```python
from build123d import *

# Parameters (mm, degrees)
F0_W     = 19.97
F0_H     = 100
F1_DEPTH = 0.6
F2_R     = 9.5
F3_R     = 2
F4_DEPTH = 0.601


with BuildPart() as f1:
    # F0 (on Front) → F1 (new body)
    with BuildSketch(Plane.XZ):
        with Locations((0, 50)):
            Rectangle(F0_W, F0_H)
        with Locations((0, -50)):
            Rectangle(F0_W, F0_H)
    extrude(amount=F1_DEPTH)

    # F2
    f2_edges = [f1.edges().sort_by_distance(p)[0] for p in [
        (9.985, -0.3, 100),
        (-9.985, -0.3, 100),
        (9.985, -0.3, -100),
        (-9.985, -0.3, -100),
    ]]
    fillet(f2_edges, radius=F2_R)

    # F3 (on face) → F4 (cut, through all)
    with BuildSketch(Plane.XZ.offset(0.6)):
        with Locations((0, 90.5)):
            Circle(F3_R)
        with Locations((0, -90.5)):
            Circle(F3_R)
    extrude(amount=-F4_DEPTH, mode=Mode.SUBTRACT)


solid = f1.part
```
Could you check a few things on this model? Use its own coordinates, in mm. Coordinates: 2 decimals unless noted, no trailing zeros. Order: outer loops, then holes, each group sorted by start corner. A loop starts at its lowest first (then second) coordinate and runs counter-clockwise, first axis right, second up. Notation, with made-up numbers: M 77.25,38 L 106.25,38 A20 ccw 106.25,72 Z; hole C 80.25,65 d11. An arc over 180 degrees is marked long. Use a Markdown table: item, result. Add a question column.
Q1. I want a section at B-B on x = -6. List the corners of the cut face in (y, z) for me, then the cut area to 3 significant figures.
Q2. I want a section at A-A on y = -0.2. List the corners of the cut face in (x, z) for me (3 decimals).
Q3. We'd pull the mould along X, two halves only. Please class faces 1 (the cylindrical face through (7.28, -0.3, 97.14)), 2 (the cylindrical face through (-0.26, -0.304, 92.483)), 3 (the cylindrical face through (-0.26, -0.304, -88.517)), 4 (the cylindrical face through (-7.28, -0.3, 97.14)): pulls with the +X half, pulls with the -X half, needs draft (parallel to the pull), parting line crosses it, or undercut.
Q4. I want a section at C-C on x = 6.75. List the corners of the cut face in (y, z) for me, then the cut area to 3 significant figures.
Q5. If I drill on L1, parallel to Z at x = -1.25, y = -0.15; L2, parallel to Z at x = -3.5, y = -0.15; L3, parallel to Z at x = 5.25, y = -0.35, over which ranges is the centre line in solid material (lowest first)?
Checked values:
| question | item | result |
|---|---|---|
| 1 | outline | M -0.6,-98.24 L 0,-98.24 L 0,98.24 L -0.6,98.24 Z |
| 1 | area | 118 mm² |
| 2 | outline | M -9.985,-90.5 A9.5 ccw -0.485,-100 L 0.485,-100 A9.5 ccw 9.985,-90.5 L 9.985,90.5 A9.5 ccw 0.485,100 L -0.485,100 A9.5 ccw -9.985,90.5 Z; hole C 0,-90.5 d4; hole C 0,90.5 d4 |
| 3 | face 1 | pulls with the +X half |
| 3 | face 2 | undercut |
| 3 | face 3 | undercut |
| 3 | face 4 | pulls with the -X half |
| 4 | outline | M -0.6,-97.64 L 0,-97.64 L 0,97.64 L -0.6,97.64 Z |
| 4 | area | 117 mm² |
| 5 | L1 | -99.97 to -92.06, -88.94 to 88.94, 92.06 to 99.97 |
| 5 | L2 | -99.51 to 99.51 |
| 5 | L3 | -98.72 to 98.72 |
